from build123d import *

# Parameters (mm, degrees)
SKETCH1_W                       = 112
SKETCH1_H                       = 35.5
BOSS_EXTRUDE1_DEPTH             = 1
SKETCH2_W                       = 6
SKETCH2_H                       = 6
BOSS_EXTRUDE2_DEPTH             = 2
SKETCH3_R                       = 1.1
CUT_EXTRUDE1_DEPTH              = 4
SKETCH4_R                       = 2
CUT_EXTRUDE2_DEPTH              = 2
CUT_EXTRUDE3_DEPTH              = 0.2
SKETCH6_W                       = 2.2
SKETCH6_H                       = 2.2
CUT_EXTRUDE4_DEPTH              = 0.2
MIRROR2_COPY_1_DEPTH            = 0.2
MIRROR2_COPY_2_SKETCH_W         = 2.2
MIRROR2_COPY_2_SKETCH_H         = 2.2
MIRROR2_COPY_2_DEPTH            = 0.2
SKETCH7_W                       = 0.4
SKETCH7_H                       = 35.5
CUT_EXTRUDE5_DEPTH              = 4
AUFSATZ_LINEAR_AUSTRAGEN2_DEPTH = 2
VERRUNDUNG1_R                   = 2


with BuildPart() as part:
    # Sketch1 → Boss-Extrude1 (new body)
    with BuildSketch(Plane.XY):
        Rectangle(SKETCH1_W, SKETCH1_H)
    extrude(amount=BOSS_EXTRUDE1_DEPTH)

    # Sketch2 → Boss-Extrude2 (add)
    with BuildSketch(Plane.XY.offset(1)):
        with Locations((-53, 14.75)):
            Rectangle(SKETCH2_W, SKETCH2_H)
        with Locations((-53, -14.75)):
            Rectangle(SKETCH2_W, SKETCH2_H)
        with Locations((53, -14.75)):
            Rectangle(SKETCH2_W, SKETCH2_H)
        with Locations((53, 14.75)):
            Rectangle(SKETCH2_W, SKETCH2_H)
    extrude(amount=BOSS_EXTRUDE2_DEPTH)

    # Sketch3 → Cut-Extrude1 (cut, through all)
    with BuildSketch(Plane.XY.offset(3)):
        with Locations((-53, 14.75)):
            Circle(SKETCH3_R)
        with Locations((-53, -14.75)):
            Circle(SKETCH3_R)
        with Locations((53, -14.75)):
            Circle(SKETCH3_R)
        with Locations((53, 14.75)):
            Circle(SKETCH3_R)
    extrude(amount=-CUT_EXTRUDE1_DEPTH, mode=Mode.SUBTRACT)

    # Sketch4 → Cut-Extrude2 (cut)
    with BuildSketch(Plane(origin=(0, 0, 0), x_dir=(-1, 0, 0), z_dir=(0, 0, -1))):
        with Locations((-53, 14.75)):
            Circle(SKETCH4_R)
        with Locations((-53, -14.75)):
            Circle(SKETCH4_R)
        with Locations((53, 14.75)):
            Circle(SKETCH4_R)
        with Locations((53, -14.75)):
            Circle(SKETCH4_R)
    extrude(amount=-CUT_EXTRUDE2_DEPTH, mode=Mode.SUBTRACT)

    # Sketch5 → Cut-Extrude3 (cut)
    with BuildSketch(Plane(origin=(0, 0, 2), x_dir=(-1, 0, 0), z_dir=(0, 0, -1))):
        with BuildLine():
            Line((-54.1, 13.079670691), (-54.1, 16.420329309))
            ThreePointArc((-54.1, 16.420329309), (-53, 16.75), (-51.9, 16.420329309))
            Line((-51.9, 16.420329309), (-51.9, 13.079670691))
            ThreePointArc((-51.9, 13.079670691), (-53, 12.75), (-54.1, 13.079670691))
        make_face()
    cut_extrude3 = extrude(amount=-CUT_EXTRUDE3_DEPTH, mode=Mode.SUBTRACT)

    # Sketch6 → Cut-Extrude4 (cut)
    with BuildSketch(Plane(origin=(0, 0, 2.2), x_dir=(-1, 0, 0), z_dir=(0, 0, -1))):
        with Locations((-53, 14.75)):
            Rectangle(SKETCH6_W, SKETCH6_H)
    cut_extrude4 = extrude(amount=-CUT_EXTRUDE4_DEPTH, mode=Mode.SUBTRACT)

    # Mirror1: Cut-Extrude3, Cut-Extrude4 across plane
    add(cut_extrude3.mirror(Plane(origin=(0, 0, 0), x_dir=(0, 0, 1), z_dir=(1, 0, 0))), mode=Mode.SUBTRACT)
    add(cut_extrude4.mirror(Plane(origin=(0, 0, 0), x_dir=(0, 0, 1), z_dir=(1, 0, 0))), mode=Mode.SUBTRACT)

    # Mirror2: Cut-Extrude3, Cut-Extrude4 across plane
    add(cut_extrude3.mirror(Plane.ZX), mode=Mode.SUBTRACT)
    add(cut_extrude4.mirror(Plane.ZX), mode=Mode.SUBTRACT)

    # Mirror2 copy 1 sketch → Mirror2 copy 1 (cut)
    with BuildSketch(Plane(origin=(0, 0, 2), x_dir=(1, 0, 0), z_dir=(0, 0, -1))):
        with BuildLine():
            Line((-54.1, 13.079670691), (-54.1, 16.420329309))
            ThreePointArc((-54.1, 16.420329309), (-53, 16.75), (-51.9, 16.420329309))
            Line((-51.9, 16.420329309), (-51.9, 13.079670691))
            ThreePointArc((-51.9, 13.079670691), (-53, 12.75), (-54.1, 13.079670691))
        make_face()
    extrude(amount=-MIRROR2_COPY_1_DEPTH, mode=Mode.SUBTRACT)

    # Mirror2 copy 2 sketch → Mirror2 copy 2 (cut)
    with BuildSketch(Plane(origin=(0, 0, 2.2), x_dir=(1, 0, 0), z_dir=(0, 0, -1))):
        with Locations((-53, 14.75)):
            Rectangle(MIRROR2_COPY_2_SKETCH_W, MIRROR2_COPY_2_SKETCH_H)
    extrude(amount=-MIRROR2_COPY_2_DEPTH, mode=Mode.SUBTRACT)

    # Sketch7 → Cut-Extrude5 (cut, through all)
    with BuildSketch(Plane(origin=(0, 0, 0), x_dir=(-1, 0, 0), z_dir=(0, 0, -1))):
        with Locations((-55.8, 0)):
            Rectangle(SKETCH7_W, SKETCH7_H)
        with Locations((55.8, 0)):
            Rectangle(SKETCH7_W, SKETCH7_H)
    extrude(amount=-CUT_EXTRUDE5_DEPTH, mode=Mode.SUBTRACT)

    # Skizze5 → Aufsatz-Linear austragen2 (add)
    with BuildSketch(Plane.XY.offset(1)):
        Polygon((-50, 11.75), (0, 0), (50, 11.75), (55.6, 11.75), (55.6, 9.984275645), (6.55686033, -1.540862177), (50, -11.75), (50, -14.831724355), (0, -3.081724355), (-50, -14.831724355), (-50, -11.75), (-6.55686033, -1.540862177), (-55.6, 9.984275645), (-55.6, 11.75), align=None)
    extrude(amount=AUFSATZ_LINEAR_AUSTRAGEN2_DEPTH)

    # Verrundung1
    verrundung1_edges = [part.edges().sort_by_distance(p)[0] for p in [
        (-6.55686033, -1.540862177, 2),
        (0, -3.081724355, 2),
        (6.55686033, -1.540862177, 2),
        (0, 0, 2),
    ]]
    fillet(verrundung1_edges, radius=VERRUNDUNG1_R)


solid = part.part
CAD build for the part. Positions are in the model's coordinates, mm. A direction names the side the tool comes from. Give positions to 0.01 mm unless a question says otherwise; leave off trailing zeros. Write each loop counter-clockwise with the first axis right and the second up, starting at its lowest first coordinate (ties: lowest second). Pieces come first, ordered by that corner, then holes. Notation, with made-up numbers: M 39,42.5 L 49,42.5 A33 ccw 49,76.5 Z; hole C 69,62 d11. An arc over 180 degrees is marked long. Put each result on its own line as item: value. Start each with the question number.
(1) Which spindle directions (+Z, -Z, +X, -X, +Y, -Y) get a long thin tool onto all of the face, cutting with end or side? Do faces 4 (the face through (-32.667, -7.677, 1.986)), 5 (the face through (53, -11.75, 2)), 6 (the face through (50, -16, 2)), 7 (the face through (-1, 11, 1)). Say none if no direction does.
(2) Band-saw the part on B-B, the plane x = 5. Write the cut outline in (y, z) (3 decimals).
(3) Band-saw the part on C-C, the plane x = -23.5. Write the cut outline in (y, z).
(4) Band-saw the part on D-D, the plane y = 5. Write the cut outline in (x, z).
(5) Flat gauge pins, fed straight in: pin 1 Ø1 at (x, z) = (10.5, 2) entering from +Y (3 decimals); pin 2 Ø2.5 at (x, y) = (53, -14.75) entering from -Z; pin 3 Ø8 at (x, y) = (1, 6) entering from +Z; pin 4 Ø12 at (x, y) = (31.5, 2.5) entering from +Z. Where does each tip first touch, or does it go through?
(6) Probe L1, parallel to X at y = -14.75, z = 0.65; L2, parallel to Y at x = 53, z = 0.55; L3, parallel to X at y = 14.75, z = 2.8. List the from-to ranges inside material, lowest first.
(7) Band-saw the part on A-A, the plane y = -1. Write the cut outline in (x, z), and give its area (3 significant figures).
(8) Mould opens along X. For faces 1 (the face through (-53.87, 14.08, 2.7)), 2 (the face through (35.506, 5.262, 1.986)), 3 (the face through (-53, -11.75, 2)) say: +X half, -X half, draft (parallel to the pull), parting line (faces both ways), or undercut.
Response values:
1. face 4: +Z, -X
1. face 5: +Z, +X
1. face 6: +Z, -Y
1. face 7: +Z, +Y
2. outline: M -17.75,0 L 17.75,0 L 17.75,1 L 1.175,1 L 1.175,3 L -4.257,3 L -4.257,1 L -17.75,1 Z
3. outline: M -17.75,0 L 17.75,0 L 17.75,1 L 5.52,1 L 5.52,3 L 2.44,3 L 2.44,1 L -5.52,1 L -5.52,3 L -8.6,3 L -8.6,1 L -17.75,1 Z
4. outline: M -55.6,0 L 55.6,0 L 55.6,1 L 34.39,1 L 34.39,3 L 21.28,3 L 21.28,1 L -21.28,1 L -21.28,3 L -34.39,3 L -34.39,1 L -55.6,1 Z
5. pin 1: stops at y = 2.585
5. pin 2: stops at z = 2
5. pin 3: stops at z = 1
5. pin 4: stops at z = 3
6. L1: x = -55.6 to -55, -51 to 51, 55 to 55.6
6. L2: y = -17.75 to -16.75, -12.75 to 12.75, 16.75 to 17.75
6. L3: x = -55.6 to -54.1, -51.9 to -50, 50 to 51.9, 54.1 to 55.6
7. outline: M -55.6,0 L 55.6,0 L 55.6,1 L 13.37,1 L 13.37,3 L -13.37,3 L -13.37,1 L -55.6,1 Z
7. area: 165 mm2
8. face 1: undercut
8. face 2: +X half
8. face 3: draft
